Source: CAD feature listing. Evaluate the final solid. Frame: model axes, mm. A direction names the side the tool comes from. Give positions to 0.01 mm unless a question says otherwise; leave off trailing zeros. Write each loop counter-clockwise with the first axis right and the second up, starting at its lowest first coordinate (ties: lowest second). Pieces come first, ordered by that corner, then holes. Notation, with made-up numbers: (30, 61.25) - (63, 61.25) arc R17 cw to (63, 67.25) - close; hole circle Ø3 at (-17.5, 88). An arc over 180 degrees is marked (long way). One line per question, with ' | ' between items. Start each with the question number.
(1) Section D-D, the plane z = 10.25. Return loops of the section in (x, y).
(2) Ray query, line 1 (Y direction, x = -19.8, z = 6); line 2 (X direction, y = -29.8, z = 15); line 3 (Y direction, x = 19.5, z = 9). Return the intervals inside material, ascending. Write a range as [from, to].
(3) Section B-B, the plane y = -29. Return loops of the section in (x, z).
(4) Pin query (flat end, axial travel): pin 1 (5 mm diameter, centred on y = 1, z = 16.5, fed in from +X). Return the tip coordinate at first contact, or that it passes through.
(5) Draft query along Y for faces 4 (the flat face through (0, 34.1, 15)), 5 (the flat face through (-20, 0, 30)), 6 (the cylindrical face through (-20.958, -10.735, 5.772)), 7 (the flat face through (3, -28.1, 12)). Return one class per face: +Y half, -Y half, draft (parallel to the pull), parting line (faces both ways), or undercut.
(6) Section C-C, the plane y = 9. Return loops of the section in (x, z).
(7) Access query for faces 1 (the flat face through (-18, 0, 15)), 2 (the flat face through (-20, 0, 0)), 3 (the cylindrical face through (18, -31, 15)). Directions: +Z, -Z, +X, -X, +Y, -Y. A direction counts if a zero-diameter tool reaches every point of the face in a straight line with its end or side. Return the directions, or none.
(8) Section A-A, the plane x = 19. Return loops of the section in (y, z), plus the area to 3 significant figures.
```python
from build123d import *

# Parameters (mm, degrees)
SKETCH1_W           = 48
SKETCH1_H           = 68.2
BOSS_EXTRUDE1_DEPTH = 30
SKETCH2_W           = 42
SKETCH2_H           = 56.2
CUT_EXTRUDE1_DEPTH  = 52.369348838
SKETCH4_R           = 4
SKETCH4_R_2         = 1.75
CUT_EXTRUDE3_DEPTH  = 30
SKETCH5_R           = 2.2
CUT_EXTRUDE4_DEPTH  = 30
SKETCH6_R           = 1.75
CUT_EXTRUDE5_DEPTH  = 62.861215636


with BuildPart() as part:
    # Sketch1 → Boss-Extrude1 (new body)
    with BuildSketch(Plane.XY):
        Rectangle(SKETCH1_W, SKETCH1_H)
    extrude(amount=BOSS_EXTRUDE1_DEPTH)

    # Sketch2 → Cut-Extrude1 (cut, through all)
    with BuildSketch(Plane.XY.offset(30)):
        with Locations((3, 0)):
            Rectangle(SKETCH2_W, SKETCH2_H)
    extrude(amount=-CUT_EXTRUDE1_DEPTH, mode=Mode.SUBTRACT)

    # Sketch4 → Cut-Extrude3 (cut)
    with BuildSketch(Plane.XZ.offset(34.1)):
        with Locations(Location((9, 15, 0), (0, 0, 270))):
            Circle(SKETCH4_R)
        with Locations(Location((9, 22.25, 0), (0, 0, 270))):
            Circle(SKETCH4_R_2)
        with Locations(Location((16.25, 15, 0), (0, 0, 270))):
            Circle(SKETCH4_R_2)
        with Locations(Location((9, 7.75, 0), (0, 0, 270))):
            Circle(SKETCH4_R_2)
        with Locations(Location((1.75, 15, 0), (0, 0, 270))):
            Circle(SKETCH4_R_2)
    extrude(amount=-CUT_EXTRUDE3_DEPTH, mode=Mode.SUBTRACT)

    # Sketch5 → Cut-Extrude4 (cut)
    with BuildSketch(Plane(origin=(0, 34.1, 0), x_dir=(1, 0, 0), z_dir=(0, 1, 0))):
        with Locations(Location((9, -15, 0), (0, 0, 270))):
            Circle(SKETCH5_R)
    extrude(amount=-CUT_EXTRUDE4_DEPTH, mode=Mode.SUBTRACT)

    # Sketch6 → Cut-Extrude5 (cut, through all)
    with BuildSketch(Plane(origin=(-18, 0, 0), x_dir=(0, 0, -1), z_dir=(1, 0, 0))):
        with Locations((-24, -9)):
            Circle(SKETCH6_R)
        with Locations(Location((-6, -9, 0), (0, 0, 180))):
            Circle(SKETCH6_R)
        with Locations((-6, 9)):
            Circle(SKETCH6_R)
        with Locations(Location((-24, 9, 0), (0, 0, 180))):
            Circle(SKETCH6_R)
    extrude(amount=-CUT_EXTRUDE5_DEPTH, mode=Mode.SUBTRACT)


solid = part.part
```
Check sheet entries:
1) outline: (-24, -34.1) - (24, -34.1) - (24, -28.1) - (-18, -28.1) - (-18, 28.1) - (24, 28.1) - (24, 34.1) - (-24, 34.1) - close
2) line 1: [-34.1, -10.75], [-7.25, 7.25], [10.75, 34.1] | line 2: [-24, 0], [3.5, 5], [13, 14.5], [18, 24] | line 3: [-34.1, -28.1], [28.1, 34.1]
3) outline: (-24, 0) - (24, 0) - (24, 30) - (-24, 30) - close; hole circle Ø3.5 at (1.75, 15); hole circle Ø8 at (9, 15); hole circle Ø3.5 at (9, 7.75); hole circle Ø3.5 at (9, 22.25); hole circle Ø3.5 at (16.25, 15)
4) pin 1: x = -18
5) face 4: +Y half | face 5: draft | face 6: undercut | face 7: undercut
6) outline: (-24, 0) - (-18, 0) - (-18, 4.25) - (-24, 4.25) - close; (-24, 7.75) - (-18, 7.75) - (-18, 22.25) - (-24, 22.25) - close; (-24, 25.75) - (-18, 25.75) - (-18, 30) - (-24, 30) - close
7) face 1: +Z, -Z, +X | face 2: -Z, +X, -X, +Y, -Y | face 3: -Y
8) outline: (-34.1, 0) - (-28.1, 0) - (-28.1, 30) - (-34.1, 30) - close; (28.1, 0) - (34.1, 0) - (34.1, 30) - (28.1, 30) - close | area: 360 mm²
